```python
from build123d import *

# Parameters (mm, degrees)
F0_W      = 20
F0_H      = 20
F0_R      = 1.375
F0_W_2    = 10
F0_H_2    = 15
F1_DEPTH  = 5
F3_DEPTH  = 7.125
F6_DEPTH  = 7.125
F8_DEPTH  = 1
F10_DEPTH = 1
F11_R     = 12
F12_DEPTH = 5


with BuildPart() as f1:
    # F0 (on Top) → F1 (new body)
    with BuildSketch(Plane.XY):
        with Locations((10, 10)):
            Rectangle(F0_W, F0_H)
        with Locations((2.5, 2.5)):
            Circle(F0_R, mode=Mode.SUBTRACT)
        with Locations((17.5, 2.5)):
            Circle(F0_R, mode=Mode.SUBTRACT)
        with Locations((2.5, 17.5)):
            Circle(F0_R, mode=Mode.SUBTRACT)
        with Locations((10, 10)):
            Rectangle(F0_W_2, F0_H_2, mode=Mode.SUBTRACT)
        with Locations((17.5, 17.5)):
            Circle(F0_R, mode=Mode.SUBTRACT)
    extrude(amount=F1_DEPTH)

    # F2 (on face) → F3 (join)
    with BuildSketch(Plane(origin=(0, 0, 0), x_dir=(0, -1, 0), z_dir=(-1, 0, 0))):
        with BuildLine():
            ThreePointArc((-18.5176654665, 5), (-20.379255435, 8.2822477738), (-21.025, 12))
            Line((-21.025, 12), (-24.025, 12))
            Line((-24.025, 12), (-24.025, 0))
            Line((-24.025, 0), (-20, 0))
            Line((-20, 0), (-20, 5))
            Line((-20, 5), (-18.5176654665, 5))
        make_face()
        with BuildLine():
            ThreePointArc((-1.4823345335, 5), (-10, 0.975), (-18.5176654665, 5))
            Line((-18.5176654665, 5), (-20, 5))
            Line((-20, 5), (-20, 0))
            Line((-20, 0), (0, 0))
            Line((0, 0), (0, 5))
            Line((0, 5), (-1.4823345335, 5))
        make_face()
        with BuildLine():
            ThreePointArc((1.025, 12), (0.379255435, 8.2822477738), (-1.4823345335, 5))
            Line((-1.4823345335, 5), (0, 5))
            Line((0, 5), (0, 0))
            Line((0, 0), (4.025, 0))
            Line((4.025, 0), (4.025, 12))
            Line((4.025, 12), (1.025, 12))
        make_face()
    extrude(amount=F3_DEPTH)

    # F5 (on face) → F6 (join)
    with BuildSketch(Plane.YZ.offset(20)):
        with BuildLine():
            Line((0, 5), (1.4823345335, 5))
            ThreePointArc((1.4823345335, 5), (-0.379255435, 8.2822477738), (-1.025, 12))
            Line((-1.025, 12), (-4.025, 12))
            Line((-4.025, 12), (-4.025, 0))
            Line((-4.025, 0), (0, 0))
            Line((0, 0), (0, 5))
        make_face()
        with BuildLine():
            ThreePointArc((18.5176654665, 5), (10, 0.975), (1.4823345335, 5))
            Line((1.4823345335, 5), (0, 5))
            Line((0, 5), (0, 0))
            Line((0, 0), (20, 0))
            Line((20, 0), (20, 5))
            Line((20, 5), (18.5176654665, 5))
        make_face()
        with BuildLine():
            ThreePointArc((21.025, 12), (20.379255435, 8.2822477738), (18.5176654665, 5))
            Line((18.5176654665, 5), (20, 5))
            Line((20, 5), (20, 0))
            Line((20, 0), (24.025, 0))
            Line((24.025, 0), (24.025, 12))
            Line((24.025, 12), (21.025, 12))
        make_face()
    extrude(amount=F6_DEPTH)

    # F7 (on face) → F8 (join)
    with BuildSketch(Plane.YZ.offset(27.125)):
        with BuildLine():
            Line((0.475, 12), (-1.025, 12))
            ThreePointArc((-1.025, 12), (10, 0.975), (21.025, 12))
            Line((21.025, 12), (19.525, 12))
            ThreePointArc((19.525, 12), (10, 2.475), (0.475, 12))
        make_face()
        with BuildLine():
            Line((-4.025, 12), (-4.025, 0))
            Line((-4.025, 0), (24.025, 0))
            Line((24.025, 0), (24.025, 12))
            Line((24.025, 12), (21.025, 12))
            ThreePointArc((21.025, 12), (10, 0.975), (-1.025, 12))
            Line((-1.025, 12), (-4.025, 12))
        make_face()
    extrude(amount=F8_DEPTH)

    # F9 (on face) → F10 (join)
    with BuildSketch(Plane(origin=(-7.125, 0, 0), x_dir=(0, -1, 0), z_dir=(-1, 0, 0))):
        with BuildLine():
            Line((-19.525, 12), (-21.025, 12))
            ThreePointArc((-21.025, 12), (-10, 0.975), (1.025, 12))
            Line((1.025, 12), (-0.475, 12))
            ThreePointArc((-0.475, 12), (-10, 2.475), (-19.525, 12))
        make_face()
        with BuildLine():
            Line((-21.025, 12), (-24.025, 12))
            Line((-24.025, 12), (-24.025, 0))
            Line((-24.025, 0), (4.025, 0))
            Line((4.025, 0), (4.025, 12))
            Line((4.025, 12), (1.025, 12))
            ThreePointArc((1.025, 12), (-10, 0.975), (-21.025, 12))
        make_face()
    extrude(amount=F10_DEPTH)

    # F11 (on offset) → F12 (cut, symmetric)
    with BuildSketch(Plane.YZ.offset(10)):
        with Locations((10, 12)):
            Circle(F11_R)
    extrude(amount=F12_DEPTH, both=True, mode=Mode.SUBTRACT)


solid = f1.part
```
The model under review builds one solid part; all positions refer to its coordinate system, in mm. A direction names the side the tool comes from. Coordinates: 2 decimals unless noted, no trailing zeros. Write each loop counter-clockwise with the first axis right and the second up, starting at its lowest first coordinate (ties: lowest second). Pieces come first, ordered by that corner, then holes. Notation, with made-up numbers: (-21.75, 71.25) -> (25.25, 71.25) arc R14 cw to (25.25, 96.25) -> close; hole circle Ø5 at (87.25, 74). An arc over 180 degrees is marked (long way). One line per item, written item: value. Start each with the question number.
Q1. Add section A-A, the plane y = 10. Give the boundary of the cut face in (x, z) (3 decimals), then the cut area to 3 significant figures.
Q2. For faces 1 (the face through (10, 20, 2)), 2 (the face through (-4, -2, 12)), 3 (the face through (10.07, 1.28, 3.756)), list the 3-axis set-ups (+Z, -Z, +X, -X, +Y, -Y) from which the entire face can be reached by the end or side of a thin tool; tool diameter is ignored.
Q3. To check wall thickness, follow probe 1 along Y at (x, z) = (17.5, 2) (3 decimals); probe 2 along X at (y, z) = (-2, 5.75) (3 decimals); probe 3 along X at (y, z) = (0.5, 7) (3 decimals). State the ranges of each line that lie inside material, in increasing order.
Q4. Add section C-C, the plane x = 11.5. Give the boundary of the cut face in (y, z).
Q5. Add section B-B, the plane x = 2.5. Give the boundary of the cut face in (y, z) (3 decimals).
Q6. Clearance check with flat-ended pins moving along their axes: P1, Ø6, axis at x = 6, y = 7, coming from the +Z side; P2, Ø1.5, axis at x = 12, z = 1.5, coming from the -Y side; P3, Ø5, axis at x = 9.5, z = 6.5, coming from the +Y side. State where each tip first meets the part, or that it passes through.
Q7. Add section D-D, the plane z = 7.5. Give the boundary of the cut face in (x, y) (3 decimals).
Q8. The part is to be moulded in two halves that separate along X. For faces 4 (the face through (16.126, 2.56, 2.465)), 5 (the face through (27.618, 10.209, 2.477)), 6 (the face through (-8.125, 10, 2)), say which applies: +X half, -X half, draft (parallel to the pull), parting line (faces both ways), or undercut.
Response:
1. outline: (-8.125, 0) -> (5, 0) -> (5, 5) -> (0, 5) -> (0, 0.975) -> (-7.125, 0.975) -> (-7.125, 2.475) -> (-8.125, 2.475) -> close; (15, 0) -> (28.125, 0) -> (28.125, 2.475) -> (27.125, 2.475) -> (27.125, 0.975) -> (20, 0.975) -> (20, 5) -> (15, 5) -> close
1. area: 68.8 mm²
2. face 1: +Z, -Z, +Y
2. face 2: +Z, +X, -X, +Y, -Y
2. face 3: +Z
3. probe 1: 0 to 1.125, 3.875 to 16.125, 18.875 to 20
3. probe 2: -8.125 to 0, 20 to 28.125
3. probe 3: -8.125 to -7.125, 27.125 to 28.125
4. outline: (0, 0) -> (2.5, 0) -> (2.5, 2.63) arc R12 cw to (0.25, 5) -> (0, 5) -> close; (17.5, 0) -> (20, 0) -> (20, 5) -> (19.75, 5) arc R12 cw to (17.5, 2.63) -> close
5. outline: (0, 0) -> (1.125, 0) -> (1.125, 5) -> (0, 5) -> close; (3.875, 0) -> (16.125, 0) -> (16.125, 5) -> (3.875, 5) -> close; (18.875, 0) -> (20, 0) -> (20, 5) -> (18.875, 5) -> close
6. P1: z = 5
6. P2: y = 0
6. P3: y = 20
7. outline: (-8.125, -4.025) -> (0, -4.025) -> (0, -0.065) -> (-7.125, -0.065) -> (-7.125, 1.605) -> (-8.125, 1.605) -> close; (-8.125, 18.395) -> (-7.125, 18.395) -> (-7.125, 20.065) -> (0, 20.065) -> (0, 24.025) -> (-8.125, 24.025) -> close; (20, -4.025) -> (28.125, -4.025) -> (28.125, 1.605) -> (27.125, 1.605) -> (27.125, -0.065) -> (20, -0.065) -> close; (20, 20.065) -> (27.125, 20.065) -> (27.125, 18.395) -> (28.125, 18.395) -> (28.125, 24.025) -> (20, 24.025) -> close
8. face 4: undercut
8. face 5: draft
8. face 6: -X half
